Job drawing, mm, ordinate dimensions from the low corner. One solid piece. A direction names the side the tool comes from. Round coordinates to 2 decimals unless told otherwise and drop trailing zeros. Order: outer loops, then holes, each group sorted by start corner. A loop starts at its lowest first (then second) coordinate and runs counter-clockwise, first axis right, second up. Notation, with made-up numbers: (-14, 48.5) -> (-4, 48.5) arc R11 cw to (-4, 60.5) -> close; hole circle Ø10 at (5, 49). An arc over 180 degrees is marked (long way). Use CSV: the item, a comma, the result in double quotes.
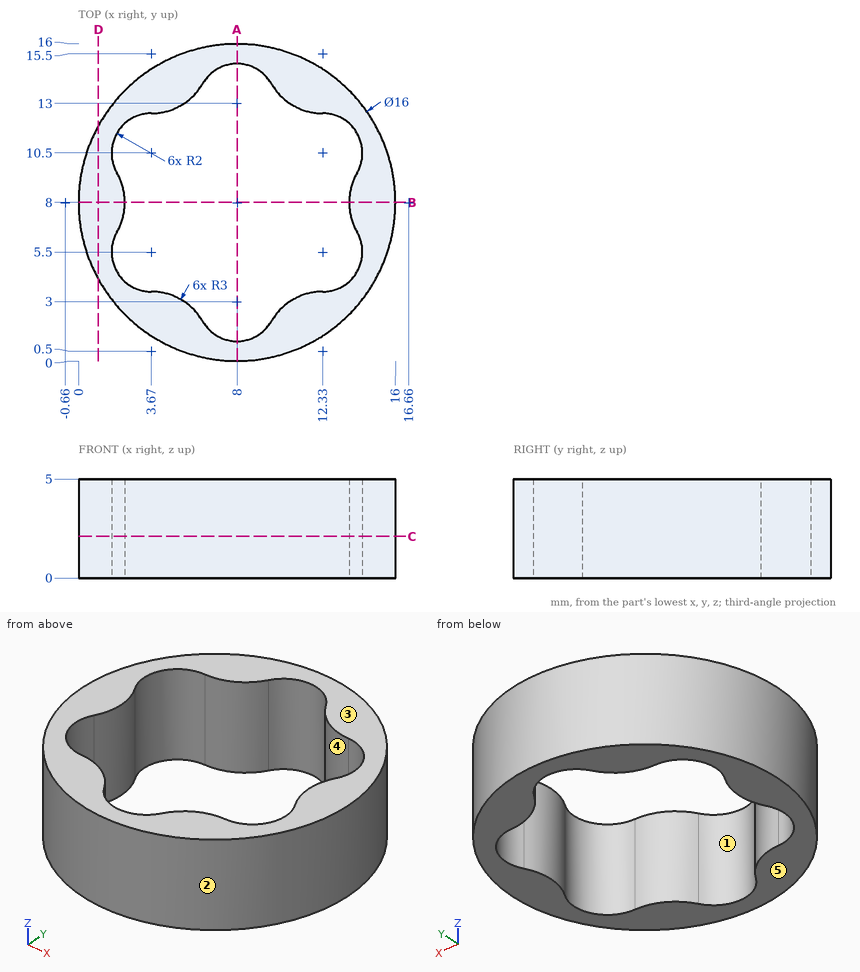
(1) Which spindle directions (+Z, -Z, +X, -X, +Y, -Y) get a long thin tool onto all of the face, cutting with end or side? Do the marked faces 4 and 5. Say none if no direction does.
Reply:
face 4,"+Z, -Z"
face 5,"-Z, +X, -X, +Y, -Y"
(2) Drop a flat-ended pin along its axis: P1, Ø1.5, axis at y = 14, z = 2, coming from the -X side. Give the stop position or say it passes through.
Reply:
P1,"x = 1.96"
(3) Probe probe 1 along Y at (x, z) = (9.75, 1.2) (1 decimal); probe 2 along Y at (x, z) = (13.5, 0.8); probe 3 along X at (y, z) = (14, 4.8). List the from-to ranges inside material, lowest first. Write a range as [from, to].
Reply:
probe 1,"[0.2, 2], [14, 15.8]"
probe 2,"[2.19, 3.88], [12.12, 13.81]"
probe 3,"[2.71, 6.27], [9.73, 13.29]"
(4) Cut at B-B, the plane y = 8. Give the cut face in (x, z), then the cut area to 3 significant figures.
Reply:
outline,"(0, 0) -> (2.34, 0) -> (2.34, 5) -> (0, 5) -> close; (13.66, 0) -> (16, 0) -> (16, 5) -> (13.66, 5) -> close"
area,"23.4 mm2"
(5) Cut at C-C, the plane z = 2.1. Give the cut face in (x, y).
Reply:
outline,"circle Ø16 at (8, 8); hole (1.94, 6.5) arc R2 ccw to (3.67, 3.5) arc R3 cw to (6.27, 2) arc R2 ccw to (9.73, 2) arc R3 cw to (12.33, 3.5) arc R2 ccw to (14.06, 6.5) arc R3 cw to (14.06, 9.5) arc R2 ccw to (12.33, 12.5) arc R3 cw to (9.73, 14) arc R2 ccw to (6.27, 14) arc R3 cw to (3.67, 12.5) arc R2 ccw to (1.94, 9.5) arc R3 cw to start"
(6) Pull direction Y, two halves, no side cores. Call the marked faces 1, 2 and 3: released by +Y, released by -Y, zero draft, split by the parting line, or undercut.
Reply:
face 1,"undercut"
face 2,"split by the parting line"
face 3,"zero draft"
(7) Cut at D-D, the plane x = 1. Give the cut face in (y, z), then the cut area to 3 significant figures.
Reply:
outline,"(4.13, 0) -> (11.87, 0) -> (11.87, 5) -> (4.13, 5) -> close"
area,"38.7 mm2"
(8) Cut at A-A, the plane x = 8. Give the cut face in (y, z), then the cut area to 3 significant figures.
Reply:
outline,"(0, 0) -> (1, 0) -> (1, 5) -> (0, 5) -> close; (15, 0) -> (16, 0) -> (16, 5) -> (15, 5) -> close"
area,"10.0 mm2"
